Build history of the part. All positions in model axes, mm. A direction names the side the tool comes from. Round coordinates to 2 decimals unless told otherwise and drop trailing zeros. Write each loop counter-clockwise with the first axis right and the second up, starting at its lowest first coordinate (ties: lowest second). Pieces come first, ordered by that corner, then holes.
from build123d import *

# Parameters (mm, degrees)
BOSS_EXTRUDE1_DEPTH = 88.9
SKETCH13_R          = 1.524
CUT_EXTRUDE1_DEPTH  = 88.9
SKETCH12_R          = 1.524
CUT_EXTRUDE2_DEPTH  = 88.9


with BuildPart() as part:
    # Sketch11 → Boss-Extrude1 (new body)
    with BuildSketch(Plane(origin=(0, 0, 0), x_dir=(0, 0, -1), z_dir=(1, 0, 0))):
        with BuildLine():
            Line((0, 0), (0, -31.09642636))
            ThreePointArc((0, -31.09642636), (-2.001946694, -36.244423742), (-6.95587324, -38.68742996))
            Line((-6.95587324, -38.68742996), (-38.1, -41.412187987))
            Line((-38.1, -41.412187987), (-38.1, -37.486427648))
            Line((-38.1, -37.486427648), (-7.28793662, -34.790721402))
            ThreePointArc((-7.28793662, -34.790721402), (-4.810973347, -33.569218294), (-3.81, -30.995219603))
            Line((-3.81, -30.995219603), (-3.81, 0))
            Line((-3.81, 0), (0, 0))
        make_face()
    extrude(amount=BOSS_EXTRUDE1_DEPTH)

    # Sketch13 → Cut-Extrude1 (cut)
    with BuildSketch(Plane.XY.offset(3.81)):
        with Locations((69.85, -15.24)):
            Circle(SKETCH13_R)
        with Locations((19.05, -15.24)):
            Circle(SKETCH13_R)
    extrude(amount=-CUT_EXTRUDE1_DEPTH, mode=Mode.SUBTRACT)

    # Sketch12 → Cut-Extrude2 (cut)
    with BuildSketch(Plane(origin=(0, -33.89367833, -2.965312619), x_dir=(1, 0, 0), z_dir=(0, 0.9961946980917459, 0.08715574274765452))):
        with Locations(Location((69.85, -25.982175442, 0), (0, 0, 270))):
            Circle(SKETCH12_R)
        with Locations(Location((19.05, -25.982175442, 0), (0, 0, 270))):
            Circle(SKETCH12_R)
    extrude(amount=-CUT_EXTRUDE2_DEPTH, mode=Mode.SUBTRACT)


solid = part.part
1) Wall check: L1, parallel to X at y = -15, z = 1; L2, parallel to Z at x = 78, y = -11; L3, parallel to Y at x = 19.05, z = 2.7. Give the ranges that are in metal, low to high.
Results:
L1: x = 0 to 17.55, 20.55 to 68.35, 71.35 to 88.9
L2: z = 0 to 3.81
L3: y = -36.92 to -16.76, -13.72 to 0
2) Slice it at B-B (x = 64.5). Write the cut outline in (y, z).
Results:
outline: (-41.41, 38.1) - (-38.69, 6.96) arc R7.62 ccw to (-31.1, 0) - (0, 0) - (0, 3.81) - (-31, 3.81) arc R3.81 cw to (-34.79, 7.29) - (-37.49, 38.1) - close
3) Slice it at C-C (y = -29.5). Write the cut outline in (x, z).
Results:
outline: (0, 0) - (88.9, 0) - (88.9, 3.81) - (0, 3.81) - close
4) Which spindle directions (+Z, -Z, +X, -X, +Y, -Y) get a long thin tool onto all of the face, cutting with end or side? Do faces 1 (the flat face through (44, -15, 0)), 2 (the flat face through (44, -16, 3.81)). Say none if no direction does.
Results:
face 1: -Z, +X, -X, +Y, -Y
face 2: +Z, +X, -X, +Y
5) Slice it at D-D (z = 17.5). Write the cut outline in (x, y).
Results:
outline: (0, -39.61) - (88.9, -39.61) - (88.9, -35.68) - (0, -35.68) - close
6) Pin check, flat tips, straight feed: pin 1 Ø10 at (y, z) = (-35.5, 24) entering from +X; pin 2 Ø2 at (x, y) = (60, -22) entering from +Z; pin 3 Ø1 at (x, y) = (51.5, -31.5) entering from +Z; pin 4 Ø8 at (x, z) = (59.5, 9) entering from +Y. Stop position of each tip, or through.
Results:
pin 1: stops at x = 88.9
pin 2: stops at z = 3.81
pin 3: stops at z = 3.94
pin 4: stops at y = -33.76
7) Mould opens along X. For faces 3 (the cylindrical face through (68.727, -14.21, 1.932)), 4 (the flat face through (88.9, -28, 3)), 5 (the flat face through (43.83, -40.03, 22.31)), 6 (the cylindrical face through (20.504, -14.782, 1.932)) say: released by +X, released by -X, zero draft, split by the parting line, or undercut.
Results:
face 3: undercut
face 4: released by +X
face 5: zero draft
face 6: undercut
8) Slice it at A-A (y = -15.24). Write the cut outline in (x, z).
Results:
outline: (0, 0) - (17.53, 0) - (17.53, 3.81) - (0, 3.81) - close; (20.57, 0) - (68.33, 0) - (68.33, 3.81) - (20.57, 3.81) - close; (71.37, 0) - (88.9, 0) - (88.9, 3.81) - (71.37, 3.81) - close
